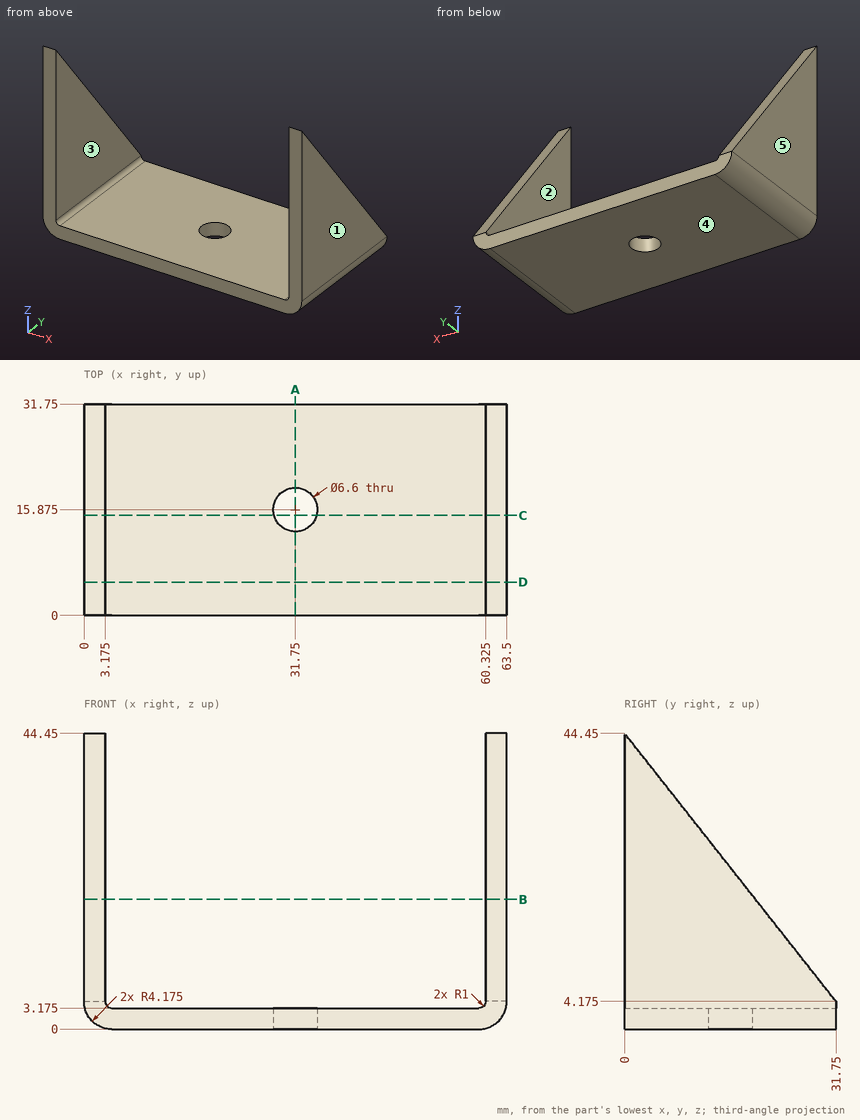
For this review, use the dimensioned drawing (mm, ordinates from the lowest corner) and the shaded views. A direction names the side the tool comes from. Round coordinates to 2 decimals unless told otherwise and drop trailing zeros. Order: outer loops, then holes, each group sorted by start corner. A loop starts at its lowest first (then second) coordinate and runs counter-clockwise, first axis right, second up. Notation, with made-up numbers: (12, -5) -> (66, -5) arc R27 cw to (66, 20) -> close; hole circle Ø4 at (43.5, 25.5). An arc over 180 degrees is marked (long way). Write item = value, one per line. Start each with the question number.
Item 1: Consider section A-A on x = 31.75. Write out the cut boundary in (y, z) (3 decimals), plus the area to 3 significant figures.
Item 2: Consider section D-D on y = 5. Write out the cut boundary in (x, z) (3 decimals), plus the area to 3 significant figures.
Item 3: Consider section B-B on z = 19.5. Write out the cut boundary in (x, y) (3 decimals).
Item 4: For the marked faces 1 and 2, list the 3-axis set-ups (+Z, -Z, +X, -X, +Y, -Y) from which the entire face can be reached by the end or side of a thin tool; tool diameter is ignored.
Item 5: For line 1 along X through (y, z) = (23, 13) (3 decimals); line 2 along Y through (x, z) = (31.75, 1.5) (3 decimals); line 3 along Z through (x, y) = (10, 15.5) (3 decimals), list the stretches that pass through material, from the lowest coordinate up.
Item 6: Clearance check with flat-ended pins moving along their axes: pin 1 Ø1 at (x, y) = (32.5, 24.5) entering from +Z (3 decimals); pin 2 Ø4 at (x, y) = (31.75, 15.875) entering from -Z. State where each tip first meets the part, or that it passes through.
Item 7: Consider section C-C on y = 15. Write out the cut boundary in (x, z) (3 decimals).
Item 8: Mouldability with a two-part tool opening along X and no side actions: class the marked faces 3, 4 and 5 as released by +X, released by -X, zero draft, split by the parting line, or undercut.
Conclusion:
q1.outline = (0, 0) -> (12.575, 0) -> (12.575, 3.175) -> (0, 3.175) -> close; (19.175, 0) -> (31.75, 0) -> (31.75, 3.175) -> (19.175, 3.175) -> close
q1.area = 79.9 mm2
q2.outline = (0, 4.175) arc R4.175 ccw to (4.175, 0) -> (59.325, 0) arc R4.175 ccw to (63.5, 4.175) -> (63.5, 38.107) -> (60.325, 38.107) -> (60.325, 4.175) arc R1 cw to (59.325, 3.175) -> (4.175, 3.175) arc R1 cw to (3.175, 4.175) -> (3.175, 38.107) -> (0, 38.107) -> close
q2.area = 416 mm2
q3.outline = (0, 0) -> (3.175, 0) -> (3.175, 19.669) -> (0, 19.669) -> close; (60.325, 0) -> (63.5, 0) -> (63.5, 19.669) -> (60.325, 19.669) -> close
q4.face_1 = +Z, -Z, +X, +Y, -Y
q4.face_2 = +Z, +Y, -Y
q5.line_1 = 0 to 3.175, 60.325 to 63.5
q5.line_2 = 0 to 12.575, 19.175 to 31.75
q5.line_3 = 0 to 3.175
q6.pin_1 = 3.175
q6.pin_2 = through
q7.outline = (0, 4.175) arc R4.175 ccw to (4.175, 0) -> (28.568, 0) -> (28.568, 3.175) -> (4.175, 3.175) arc R1 cw to (3.175, 4.175) -> (3.175, 25.422) -> (0, 25.422) -> close; (34.932, 0) -> (59.325, 0) arc R4.175 ccw to (63.5, 4.175) -> (63.5, 25.422) -> (60.325, 25.422) -> (60.325, 4.175) arc R1 cw to (59.325, 3.175) -> (34.932, 3.175) -> close
q8.face_3 = undercut
q8.face_4 = zero draft
q8.face_5 = released by -X
